from build123d import *

# Parameters (mm, degrees)
F0_R     = 42.5
F1_DEPTH = 60
F2_R     = 20
F3_DEPTH = 100
F3_TAPER = 3
F4_W     = 15
F4_H     = 15
F5_DEPTH = 50
F6_R     = 5
F7_DEPTH = 50


with BuildPart() as f1:
    # F0 (on Front) → F1 (new body, symmetric)
    with BuildSketch(Plane.XZ):
        Circle(F0_R)
    extrude(amount=F1_DEPTH, both=True)

    # F2 (on Top) → F3 (join)
    with BuildSketch(Plane.XY):
        Circle(F2_R)
    extrude(amount=-F3_DEPTH, taper=F3_TAPER)

    # F4 (on face) → F5 (cut)
    with BuildSketch(Plane(origin=(0, 0, -100), x_dir=(1, 0, 0), z_dir=(0, 0, -1))):
        Rectangle(F4_W, F4_H)
    extrude(amount=-F5_DEPTH, mode=Mode.SUBTRACT)

    # F6 (on Right) → F7 (cut)
    with BuildSketch(Plane.YZ):
        with Locations((0, -85)):
            Circle(F6_R)
    extrude(amount=-F7_DEPTH, mode=Mode.SUBTRACT)


solid = f1.part
The listing builds one solid part. Answer for the finished solid, in the listing's coordinates (mm). A direction names the side the tool comes from. Round coordinates to 2 decimals unless told otherwise and drop trailing zeros. Write each loop counter-clockwise with the first axis right and the second up, starting at its lowest first coordinate (ties: lowest second). Pieces come first, ordered by that corner, then holes. Notation, with made-up numbers: M 59.5,-5.75 L 106.5,-5.75 A18 cw 106.5,8.25 Z; hole C -23,65.5 d5. An arc over 180 degrees is marked long. Write each question's results on one line, items separated by ' | '. Start each with the question number.
Item 1: For faces 1 (the face through (-12, 3, -81)), 2 (the face through (0, 7.5, -75)), 3 (the face through (-1, -60, 1)), determine the directions among +Z, -Z, +X, -X, +Y, -Y from which every point of the face is accessible in a straight line to the end or side of a thin tool.
Item 2: For a pull along X with two mould halves and no side action, classify faces 4 (the face through (10, 0, -100)), 5 (the face through (22.848, -0.84, 35.836)), 6 (the face through (0, 0, -50)) as pulls with the +X half, pulls with the -X half, needs draft (parallel to the pull), parting line crosses it, or undercut.
Item 3: A cutting plane is placed at C-C on z = -83. Write down the section's boundary in (x, y).
Item 4: A cutting plane is placed at D-D on y = -42.5. Write down the section's boundary in (x, z).
Item 5: A cutting plane is placed at B-B on z = -66.5. Write down the section's boundary in (x, y), and give its area (3 significant figures).
Item 6: A cutting plane is placed at A-A on x = 0. Write down the section's boundary in (y, z).
Item 7: Straight lines are drawn through the part: L1, parallel to Z at x = -0.5, y = -39.5; L2, parallel to Z at x = -11, y = 0; L3, parallel to Y at x = -10.25, z = -85. For each, find the intervals that lie inside material, in ascending order. Write a range as [from, to].
Item 8: Flat-ended cylindrical pins translate along their axes: pin 1 Ø8 at (x, y) = (-19, 17.5) entering from +Z; pin 2 Ø4.5 at (y, z) = (2, -74.5) entering from -X; pin 3 Ø6 at (x, z) = (-6.5, -53) entering from -Y. Find the tip coordinate at first contact, or state that the pin passes through.
Check sheet entries:
1) face 1: -X | face 2: -Z | face 3: +Z, -Z, +X, -X, -Y
2) face 4: needs draft | face 5: parting line crosses it | face 6: undercut
3) outline: M -14.96,-4.58 A15.65 ccw long -14.96,4.58 L -7.5,4.58 L -7.5,7.5 L 7.5,7.5 L 7.5,-7.5 L -7.5,-7.5 L -7.5,-4.58 Z
4) outline: C 0,0 d85
5) outline: C 0,0 d33.03; hole M -7.5,-7.5 L 7.5,-7.5 L 7.5,7.5 L -7.5,7.5 Z | area: 632 mm²
6) outline: M -60,-42.5 L -17.77,-42.5 L -14.76,-100 L -7.5,-100 L -7.5,-50 L 7.5,-50 L 7.5,-100 L 14.76,-100 L 17.77,-42.5 L 60,-42.5 L 60,42.5 L -60,42.5 Z
7) L1: [-42.5, 42.5] | L2: [-100, -90], [-80, 41.05] | L3: [-11.69, -5], [5, 11.69]
8) pin 1: z = 39.76 | pin 2: x = -16.18 | pin 3: y = -16.88
